Part print with two shaded views. Sizes in mm from the minimum x, y, z corner. A direction names the side the tool comes from. Round coordinates to 2 decimals unless told otherwise and drop trailing zeros. Order: outer loops, then holes, each group sorted by start corner. A loop starts at its lowest first (then second) coordinate and runs counter-clockwise, first axis right, second up. Notation, with made-up numbers: (20, 80.5) - (36, 80.5) arc R34 cw to (36, 111.5) - close; hole circle Ø10 at (4, -9). An arc over 180 degrees is marked (long way). Use one line per item in the form item = value.
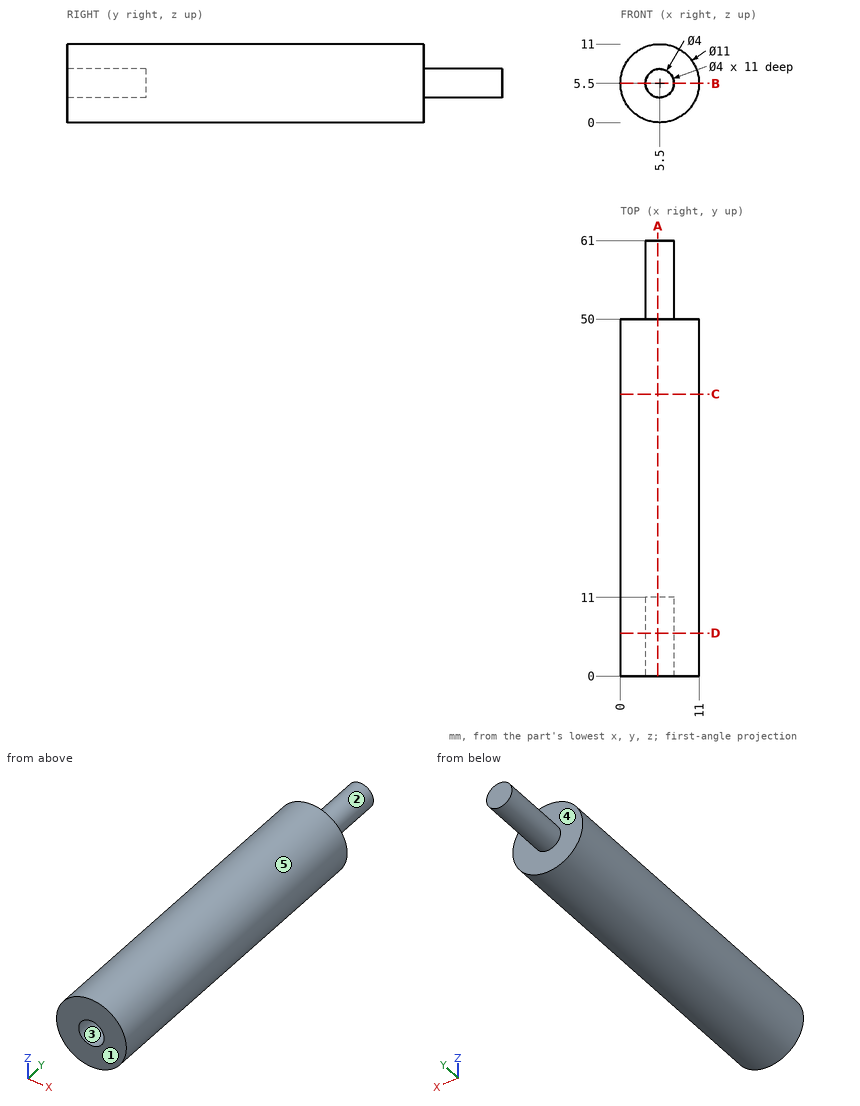
(1) Pull direction Z, two halves, no side cores. Call the marked faces 3, 4 and 5: released by +Z, released by -Z, zero draft, split by the parting line, or undercut.
Report:
face_3 = undercut
face_4 = zero draft
face_5 = split by the parting line
(2) Slice it at D-D on y = 6. Give the cut face in (x, z).
Report:
outline = circle Ø11 at (5.5, 5.5); hole circle Ø4 at (5.5, 5.5)
(3) Probe probe 1 along Z at (x, y) = (5.5, 6.75); probe 2 along Y at (x, z) = (2, 1.5); probe 3 along Z at (x, y) = (1.25, 6.5). List the from-to ranges inside material, lowest first. Write a range as [from, to].
Report:
probe_1 = [0, 3.5], [7.5, 11]
probe_2 = [0, 50]
probe_3 = [2.01, 8.99]
(4) Slice it at A-A on x = 5.25. Give the cut face in (y, z), then the cut area to 3 significant figures.
Report:
outline = (0, 0.01) - (50, 0.01) - (50, 3.52) - (61, 3.52) - (61, 7.48) - (50, 7.48) - (50, 10.99) - (0, 10.99) - (0, 7.48) - (11, 7.48) - (11, 3.52) - (0, 3.52) - close
area = 549 mm2
(5) Tool access for the marked faces 1 and 2: list every direction of +Z, -Z, +X, -X, +Y, -Y with a clear straight run to the whole face (end or side of a thin tool).
Report:
face_1 = +Z, -Z, +X, -X, -Y
face_2 = +Y
(6) Slice it at B-B on z = 5.5. Give the cut face in (x, y).
Report:
outline = (0, 0) - (3.5, 0) - (3.5, 11) - (7.5, 11) - (7.5, 0) - (11, 0) - (11, 50) - (7.5, 50) - (7.5, 61) - (3.5, 61) - (3.5, 50) - (0, 50) - close
(7) Pin check, flat tips, straight feed: pin 1 (1 mm diameter, centred on x = 8.5, y = 18, fed in from +Z); pin 2 (4.5 mm diameter, centred on x = 6, z = 6, fed in from -Y); pin 3 (3 mm diameter, centred on y = 11.5, z = 9, fed in from +X); pin 4 (2 mm diameter, centred on y = 11, z = 4, fed in from -X). Stop position of each tip, or through.
Report:
pin_1 = 10.4
pin_2 = 0
pin_3 = 10.62
pin_4 = 0.02
(8) Slice it at C-C on y = 39.5. Give the cut face in (x, z), then the cut area to 3 significant figures.
Report:
outline = circle Ø11 at (5.5, 5.5)
area = 95.0 mm2
